Work out the finished part from the listing and answer in its coordinate system (mm). A direction names the side the tool comes from. Round coordinates to 2 decimals unless told otherwise and drop trailing zeros. Order: outer loops, then holes, each group sorted by start corner. A loop starts at its lowest first (then second) coordinate and runs counter-clockwise, first axis right, second up. Notation, with made-up numbers: M -6,-16.75 L 21,-16.75 A4 ccw 21,-12.75 Z; hole C 0,-7 d3. An arc over 180 degrees is marked long. Answer as a JSON object with one key per item and string values. Group by question number.
from build123d import *

# Parameters (mm, degrees)
F1_DEPTH    = 10.16
F0_W        = 13.6915519834
F0_H        = 11.6948671639
F2_DEPTH    = 20.32
F4_DEPTH    = 77.0159752498
F5_W        = 59.2985060066
F5_H        = 8.0565831158
F6_DEPTH    = 4.5666936785
F7_T1_DEPTH = 84.5685063134
F8_R        = 2.3549546022
F9_DEPTH    = 20.321


# Not quite as in the source:
# - a fillet or chamfer that OpenCascade refuses, or shapes differently, is made with other operations: its cross-section is extruded or revolved along the edge and cut away or added


with BuildPart() as f1:
    # F0 (on Top) → F1 (new body)
    with BuildSketch(Plane.XY):
        Polygon((38.5074876249, -7.2736367583), (38.5074876249, 7.2736367583), (-38.5074876249, 7.2736367583), (-38.5074876249, -7.2736367583), (-6.8457759917, -7.2736367583), (6.8457759917, -7.2736367583), align=None)
    extrude(amount=F1_DEPTH)

    # F0 (on Top) → F2 (join)
    with BuildSketch(Plane.XY):
        with Locations((0, -13.1210703403)):
            Rectangle(F0_W, F0_H)
    extrude(amount=F2_DEPTH)

    # F3 (on face) → F4 (cut, through all)
    with BuildSketch(Plane.YZ.offset(38.5074876249)):
        Polygon((5.1769153215, 4.5666936785), (1.6501703067, 1.9309354248), (-0.9334948961, 0), (7.2736367583, 0), (7.2736367583, 4.5666936785), align=None)
    extrude(amount=-F4_DEPTH, mode=Mode.SUBTRACT)

    # F5 (on face) → F6 (join, through all)
    with BuildSketch(Plane(origin=(0, 0, 4.5666936785), x_dir=(1, 0, 0), z_dir=(0, 0, -1))):
        with Locations((0.0417931005, -1.1486237636)):
            Rectangle(F5_W, F5_H)
    extrude(amount=F6_DEPTH)

    # F7: fillet of radius 5.08 on 1 edges, made by hand

    # F7_s2 → F7_t1 (cut)
    with BuildSketch(Plane.YZ.offset(-42.2424600562)):
        with BuildLine():
            ThreePointArc((0.1229152601, 0), (3.5287047345, 1.3107828324), (5.1769153215, 4.5666936785))
            Line((5.1769153215, 4.5666936785), (5.1769153215, 0))
            Line((5.1769153215, 0), (0.1229152601, 0))
        make_face()
    extrude(amount=F7_T1_DEPTH, mode=Mode.SUBTRACT)

    # F8 (on face) → F9 (cut, through all)
    with BuildSketch(Plane.XY.offset(20.32)):
        with Locations((0, -13.4750818834)):
            Circle(F8_R)
    extrude(amount=-F9_DEPTH, mode=Mode.SUBTRACT)


solid = f1.part
Item 1: Find section B-B (z = 9.25). Give the vertices of the cut face in (x, y), and give its area (3 significant figures).
Item 2: A tool of negligible diameter and unlimited length cuts with its end or side. For faces 1 (the flat face through (-23, -7.274, 5)), 2 (the flat face through (0, -7.274, 15)), 3 (the flat face through (29.691, 3, 2)), 4 (the flat face through (-29.607, 3, 2)), from which of +Z, -Z, +X, -X, +Y, -Y can it reach the whole face along a straight path? Write none if from no direction.
Item 3: Find section D-D (x = 13). Give the vertices of the cut face in (y, z).
Item 4: Each of these flat-tipped pins is pushed along its axis until it touches: pin 1 (4 mm diameter, centred on x = 0, y = -13.48, fed in from +Z); pin 2 (6 mm diameter, centred on x = 7.5, z = 16, fed in from +Y); pin 3 (3.5 mm diameter, centred on y = -14.5, z = 10, fed in from -X); pin 4 (1.7 mm diameter, centred on x = 10.5, y = 6.5, fed in from -Z). Where does it stop, or does it pass through?
Item 5: Find section A-A (x = 0). Give the vertices of the cut face in (y, z), and give its area (3 significant figures).
Item 6: Find section C-C (y = -12.5). Give the vertices of the cut face in (x, z), and give its area (3 significant figures).
Item 7: Consider L1, parallel to Y at x = 0, z = 16.25; L2, parallel to Y at x = 0, z = 7; L3, parallel to Z at x = 10, y = -4.5. Determine where each line is inside the solid, lowest interval first.
Responses:
{
 "1": {"outline": "M -38.51,-7.27 L -6.85,-7.27 L -6.85,-18.97 L 6.85,-18.97 L 6.85,-7.27 L 38.51,-7.27 L 38.51,7.27 L -38.51,7.27 Z; hole C 0,-13.48 d4.71", "area": "1,260 mm^2"},
 "2": {"face 1": "+Z, -Z, -X, -Y", "face 2": "+Z, +X, -X, +Y", "face 3": "-Z, +X, +Y", "face 4": "-Z, -X, +Y"},
 "3": {"outline": "M -7.27,0 L 0.12,0 A5.08 ccw 5.18,4.57 L 7.27,4.57 L 7.27,10.16 L -7.27,10.16 Z"},
 "4": {"pin 1": "passes through", "pin 2": "stops at y = -7.27", "pin 3": "stops at x = -6.85", "pin 4": "stops at z = 4.57"},
 "5": {"outline": "M -18.97,0 L -15.83,0 L -15.83,20.32 L -18.97,20.32 Z; M -11.12,0 L 0.12,0 A5.08 ccw 5.18,4.57 L 7.27,4.57 L 7.27,10.16 L -7.27,10.16 L -7.27,20.32 L -11.12,20.32 Z", "area": "275 mm^2"},
 "6": {"outline": "M -6.85,0 L -2.14,0 L -2.14,20.32 L -6.85,20.32 Z; M 2.14,0 L 6.85,0 L 6.85,20.32 L 2.14,20.32 Z", "area": "191 mm^2"},
 "7": {"L1": "y = -18.97 to -15.83, -11.12 to -7.27", "L2": "y = -18.97 to -15.83, -11.12 to 7.27", "L3": "z = 0 to 10.16"}
}
